Geometry check sheet. Reference: the model listing, model coordinates, mm. A direction names the side the tool comes from. Coordinates: 2 decimals unless noted, no trailing zeros. Order: outer loops, then holes, each group sorted by start corner. A loop starts at its lowest first (then second) coordinate and runs counter-clockwise, first axis right, second up.
```python
from build123d import *

# Parameters (mm, degrees)
SKETCH_1_R               = 9
SKETCH_1_R_2             = 4
EXTRUDE_1_DEPTH          = 20
EXTRUDE_2_DEPTH          = 1.5
EXTRUDE_2_DEPTH_BACK     = 1.5
SKETCH_2_R               = 45
CUT_EXTRUDE_2_DEPTH      = 67.708320321
CUT_EXTRUDE_2_DEPTH_BACK = 67.708320321
SKETCH_1_2_R             = 4
CUT_EXTRUDE_3_DEPTH      = 66.5
CUT_EXTRUDE_3_DEPTH_BACK = 66.5
SKETCH_3_R               = 10
EXTRUDE_3_DEPTH          = 7
EXTRUDE_3_DEPTH_BACK     = 7
SKETCH_5_R               = 45
SKETCH_5_R_2             = 35
EXTRUDE_4_DEPTH          = 6
EXTRUDE_4_DEPTH_BACK     = 6
SKETCH_6_R               = 47.5
SKETCH_6_R_2             = 45


with BuildPart() as part:
    # 스케치1 → 보스-돌출1 (new body)
    with BuildSketch(Plane.XY):
        Circle(SKETCH_1_R)
        Circle(SKETCH_1_R_2, mode=Mode.SUBTRACT)
    extrude(amount=EXTRUDE_1_DEPTH)

    # 스케치2 → 보스-돌출2 (add, two sides: drawn at the far end of the back side and taken through both)
    with BuildSketch(Plane.XY.offset(14).offset(-EXTRUDE_2_DEPTH_BACK)):
        Circle(SKETCH_2_R)
    extrude(amount=EXTRUDE_2_DEPTH + EXTRUDE_2_DEPTH_BACK)

    # 스케치1<2> → 컷-돌출2 (cut, two sides: drawn at the far end of the back side and taken through both)
    with BuildSketch(Plane.XY.offset(-CUT_EXTRUDE_2_DEPTH_BACK)):
        Circle(SKETCH_1_2_R)
    extrude(amount=CUT_EXTRUDE_2_DEPTH + CUT_EXTRUDE_2_DEPTH_BACK, mode=Mode.SUBTRACT)

    # 스케치3 → 컷-돌출3 (cut, two sides: drawn at the far end of the back side and taken through both)
    with BuildSketch(Plane.XY.offset(15.5).offset(-CUT_EXTRUDE_3_DEPTH_BACK)):
        with Locations((0, 21)):
            Circle(SKETCH_3_R)
        with Locations((19.972186842, 6.489356882)):
            Circle(SKETCH_3_R)
        with Locations((12.343490298, -16.989356882)):
            Circle(SKETCH_3_R)
        with Locations((-12.343490298, -16.989356882)):
            Circle(SKETCH_3_R)
        with Locations((-19.972186842, 6.489356882)):
            Circle(SKETCH_3_R)
    extrude(amount=CUT_EXTRUDE_3_DEPTH + CUT_EXTRUDE_3_DEPTH_BACK, mode=Mode.SUBTRACT)

    # 스케치5 → 보스-돌출3 (add, two sides: drawn at the far end of the back side and taken through both)
    with BuildSketch(Plane.XY.offset(14).offset(-EXTRUDE_3_DEPTH_BACK)):
        Circle(SKETCH_5_R)
        Circle(SKETCH_5_R_2, mode=Mode.SUBTRACT)
    extrude(amount=EXTRUDE_3_DEPTH + EXTRUDE_3_DEPTH_BACK)

    # 스케치6 → 보스-돌출4 (add, two sides: drawn at the far end of the back side and taken through both)
    with BuildSketch(Plane.XY.offset(14).offset(-EXTRUDE_4_DEPTH_BACK)):
        Circle(SKETCH_6_R)
        Circle(SKETCH_6_R_2, mode=Mode.SUBTRACT)
    extrude(amount=EXTRUDE_4_DEPTH + EXTRUDE_4_DEPTH_BACK)

    # 스케치9 → M4 여유 구멍1 (revolve, cut)
    with BuildSketch(Plane(origin=(0, 0, 5), x_dir=(0, 0, -1), z_dir=(1, 0, 0))):
        Polygon((0, 0), (0, 31.351936393), (2.25, 30), (2.25, 0), align=None)
    revolve(axis=Axis((0, -6.35, 5), (0, 1, 0)), mode=Mode.SUBTRACT)

    # 스케치12 → M4 여유 구멍2 (revolve, cut)
    with BuildSketch(Plane(origin=(0, 0, 5), x_dir=(0, 0, 1), z_dir=(0, 1, 0))):
        Polygon((0, 0), (0, 31.351936393), (2.25, 30), (2.25, 0), align=None)
    revolve(axis=Axis((-6.35, 0, 5), (1, 0, 0)), mode=Mode.SUBTRACT)


solid = part.part
```
Item 1: Thickness scan on line 1 along Y through (x, z) = (0, 13.35); line 2 along Y through (x, z) = (3, 16.25); line 3 along Z through (x, y) = (5, 0). Record the ranges inside material, lowest first.
Item 2: Tool access check on faces 4 (the face through (-28, -21, 18)), 5 (the face through (9.98, 6.93, 13.98)), 6 (the face through (-1.951, -8.786, 6.162)), 7 (the face through (6.114, -0.676, 7.146)). Record the directions out of +Z, -Z, +X, -X, +Y, -Y that give a thin tool (end or side, any length) a straight path to the whole face; none if there is none.
Item 3: Sectioned sample at A-A (z = 10.25). Record the cut outline in (x, y).
Item 4: Sectioned sample at D-D (z = 5). Record the cut outline in (x, y).
Item 5: Depth check by flat-ended pin: P1, Ø23, axis at x = 19.97, y = 6.49, coming from the +Z side; P2, Ø1, axis at x = 28, z = 9, coming from the -Y side; P3, Ø10, axis at y = 13, z = 18.5, coming from the -X side. Enter the tip coordinate at first touch or a pass-through.
Item 6: Sectioned sample at B-B (y = 21). Record the cut outline in (x, z), and give its area (3 significant figures).
Item 7: Release check for a two-part mould opening along X. For faces 1 (the face through (4, -2, 0)), 2 (the face through (20.765, -39.923, 7.493)), 3 (the face through (-3.2, -2.4, 9.9)) record: pulls with the +X half, pulls with the -X half, needs draft (parallel to the pull), parting line crosses it, or undercut.
Item 8: Sectioned sample at C-C (x = -20). Record the cut outline in (y, z), and give its area (3 significant figures).
Geometry check:
1. line 1: y = -47.5 to -4, 4 to 11, 31 to 47.5
1. line 2: y = -47.41 to -34.87, -8.49 to -2.65, 2.65 to 8.49, 34.87 to 47.41
1. line 3: z = 0 to 2.75, 7.25 to 20
2. face 4: +Z
2. face 5: +Z, -Z
2. face 6: -Z
2. face 7: none
3. outline: circle Ø95 at (0, 0); circle Ø18 at (0, 0); hole circle Ø70 at (0, 0); hole circle Ø8 at (0, 0)
4. outline: (-2.25, 3.31) - (-2.25, 8.71) arc R9 ccw (long way) to (8.71, -2.25) - (3.31, -2.25) arc R4 cw (long way) to start; (2.25, 3.31) arc R4 cw to (3.31, 2.25) - (8.71, 2.25) arc R9 ccw to (2.25, 8.71) - close
5. P1: stops at z = 15.5
5. P2: stops at y = -38.73
5. P3: stops at x = -46.82
6. outline: (-42.61, 8) - (-39.8, 8) - (-39.8, 7) - (-28, 7) - (-28, 12.5) - (-10, 12.5) - (-10, 15.5) - (-28, 15.5) - (-28, 21) - (-39.8, 21) - (-39.8, 20) - (-42.61, 20) - close; (10, 12.5) - (28, 12.5) - (28, 7) - (39.8, 7) - (39.8, 8) - (42.61, 8) - (42.61, 20) - (39.8, 20) - (39.8, 21) - (28, 21) - (28, 15.5) - (10, 15.5) - close
6. area: 506 mm2
7. face 1: needs draft
7. face 2: parting line crosses it
7. face 3: undercut
8. outline: (-43.08, 8) - (-40.31, 8) - (-40.31, 7) - (-28.72, 7) - (-28.72, 12.5) - (-23.42, 12.5) - (-23.42, 15.5) - (-28.72, 15.5) - (-28.72, 21) - (-40.31, 21) - (-40.31, 20) - (-43.08, 20) - close; (-10.56, 12.5) - (-3.51, 12.5) - (-3.51, 15.5) - (-10.56, 15.5) - close; (16.49, 12.5) - (28.72, 12.5) - (28.72, 7) - (40.31, 7) - (40.31, 8) - (43.08, 8) - (43.08, 20) - (40.31, 20) - (40.31, 21) - (28.72, 21) - (28.72, 15.5) - (16.49, 15.5) - close
8. area: 465 mm2
